Job drawing, mm, ordinate dimensions from the low corner. One solid piece. Give positions to 0.01 mm unless a question says otherwise; leave off trailing zeros. Order: outer loops, then holes, each group sorted by start corner. A loop starts at its lowest first (then second) coordinate and runs counter-clockwise, first axis right, second up.
1. Slice it at B-B on z = 3.75. List the corners of the cut face in (x, y).
2. Drop flat-ended pins along their axis: pin 1 Ø1 at (x, z) = (39, 20.5) entering from +Y; pin 2 Ø2.5 at (x, y) = (36, 36.5) entering from +Z; pin 3 Ø2.5 at (x, y) = (5, 5.35) entering from +Z; pin 4 Ø10 at (y, z) = (20.5, 4) entering from +X. Give the stop position or say it passes through.
3. Slice it at D-D on y = 36.35. List the corners of the cut face in (x, z) (1 decimal).
4. Slice it at A-A on y = 5.35. List the corners of the cut face in (x, z).
5. Probe line 1 (Y direction, x = 36, z = 7.25); line 2 (X direction, y = 5, z = 18); line 3 (X direction, y = 35.5, z = 15) (1 decimal). List the from-to ranges inside material, lowest first.
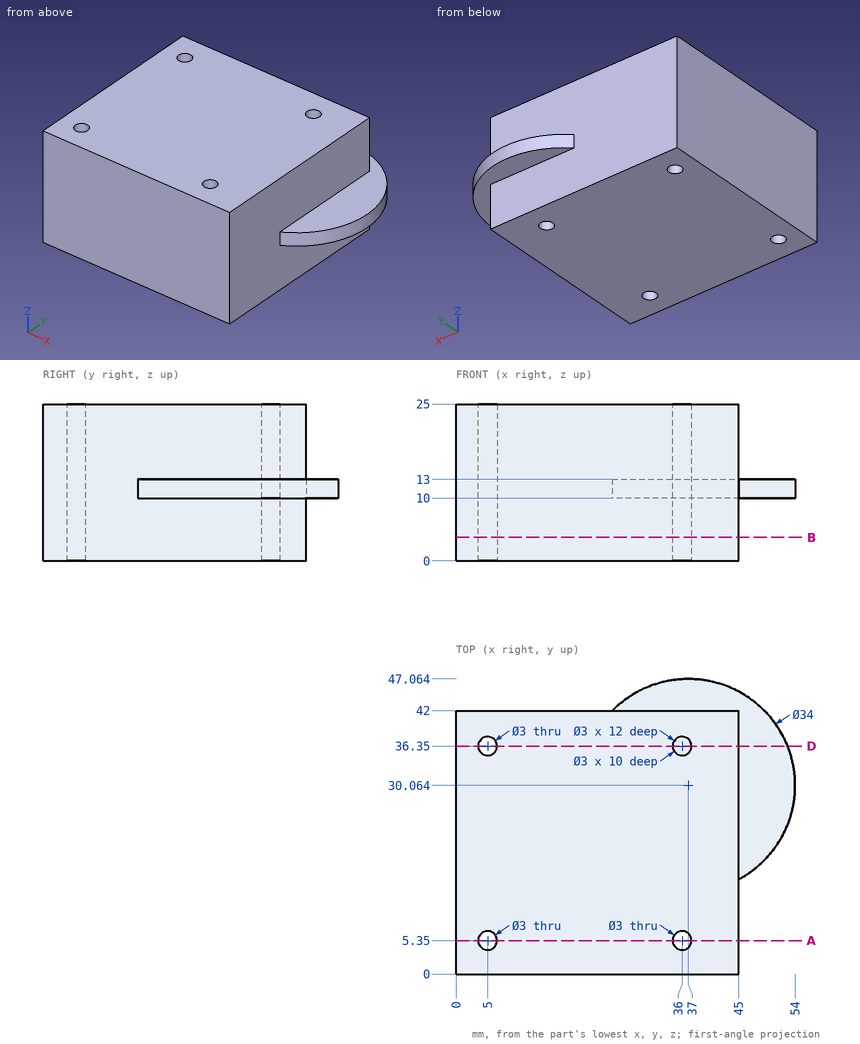
Data:
1. outline: (0, 0) - (45, 0) - (45, 42) - (0, 42) - close; hole circle Ø3 at (5, 5.35); hole circle Ø3 at (5, 36.35); hole circle Ø3 at (36, 5.35); hole circle Ø3 at (36, 36.35)
2. pin 1: stops at y = 42
2. pin 2: stops at z = 13
2. pin 3: passes through
2. pin 4: stops at x = 45
3. outline: (0, 0) - (3.5, 0) - (3.5, 25) - (0, 25) - close; (6.5, 0) - (34.5, 0) - (34.5, 10) - (37.5, 10) - (37.5, 0) - (45, 0) - (45, 10) - (52.8, 10) - (52.8, 13) - (45, 13) - (45, 25) - (37.5, 25) - (37.5, 13) - (34.5, 13) - (34.5, 25) - (6.5, 25) - close
4. outline: (0, 0) - (3.5, 0) - (3.5, 25) - (0, 25) - close; (6.5, 0) - (34.5, 0) - (34.5, 25) - (6.5, 25) - close; (37.5, 0) - (45, 0) - (45, 25) - (37.5, 25) - close
5. line 1: y = 0 to 3.85, 6.85 to 34.85, 37.85 to 42
5. line 2: x = 0 to 3.54, 6.46 to 34.54, 37.46 to 45
5. line 3: x = 0 to 3.8, 6.2 to 34.8, 37.2 to 45
